Geometry: final body of the model. Coordinates: model frame, mm. A direction names the side the tool comes from. Give positions to 0.01 mm unless a question says otherwise; leave off trailing zeros. Write each loop counter-clockwise with the first axis right and the second up, starting at its lowest first coordinate (ties: lowest second). Pieces come first, ordered by that corner, then holes. Notation, with made-up numbers: (-10.75, -9.5) - (-4.75, -9.5) arc R28 cw to (-4.75, 18.5) - close; hole circle Ø10 at (35.5, 1). An arc over 180 degrees is marked (long way). Return JSON: item names as keys, results as strings.
from build123d import *

# Parameters (mm, degrees)
SKETCH1_R               = 4
BOSS_EXTRUDE1_DEPTH     = 20
CUT_EXTRUDE1_DEPTH      = 52
CUT_EXTRUDE1_DEPTH_BACK = 35
SKETCH2_W               = 10
SKETCH2_H               = 20
SKETCH3_W               = 10
SKETCH3_H               = 10
CUT_EXTRUDE2_DEPTH      = 52
CUT_EXTRUDE3_START      = -5
CUT_EXTRUDE3_DEPTH      = 10
CUT_EXTRUDE4_START      = -5
CUT_EXTRUDE4_DEPTH      = 10
FILLET1_R               = 2
SKETCH9_R               = 4
SKETCH9_R_2             = 2.5
BOSS_EXTRUDE2_DEPTH     = 3.5
BOSS_EXTRUDE3_START     = -3.5
SKETCH10_R              = 4
SKETCH10_R_2            = 2.5
BOSS_EXTRUDE3_DEPTH     = 3.5


with BuildPart() as part:
    # Sketch1 → Boss-Extrude1 (new body)
    with BuildSketch(Plane(origin=(0, 0, 0), x_dir=(0, 0, -1), z_dir=(1, 0, 0))):
        with BuildLine():
            Line((-41.59166249, 42.046001407), (58.40833751, 42.046001407))
            add(Edge.make_bspline(
                [(58.40833751, 42.046001407), (82.40833751, 34.546001407), (58.40833751, 27.046001407)],
                knots=[0, 0, 0, 1, 1, 1], degree=2))
            Line((58.40833751, 27.046001407), (-41.59166249, 27.046001407))
            add(Edge.make_bspline(
                [(-41.59166249, 42.046001407), (-61.59166249, 34.546001407), (-41.59166249, 27.046001407)],
                knots=[0, 0, 0, 1, 1, 1], degree=2))
        make_face()
        with Locations((60.40833751, 34.546001407)):
            Circle(SKETCH1_R, mode=Mode.SUBTRACT)
    extrude(amount=BOSS_EXTRUDE1_DEPTH)

    # Sketch2 → Cut-Extrude1 (cut, two sides: drawn at the far end of the back side and taken through both)
    with BuildSketch(Plane(origin=(0, 0, 0), x_dir=(1, 0, 0), z_dir=(0, 1, 0)).offset(-CUT_EXTRUDE1_DEPTH_BACK)):
        with Locations((10, 60.40833751)):
            Rectangle(SKETCH2_W, SKETCH2_H)
    extrude(amount=CUT_EXTRUDE1_DEPTH + CUT_EXTRUDE1_DEPTH_BACK, mode=Mode.SUBTRACT)

    # Sketch3 → Cut-Extrude2 (cut)
    with BuildSketch(Plane.XZ.offset(-27.046001407)):
        with Locations((10, 46.59166249)):
            Rectangle(SKETCH3_W, SKETCH3_H)
    extrude(amount=-CUT_EXTRUDE2_DEPTH, mode=Mode.SUBTRACT)

    # Sketch4 → Cut-Extrude3 (cut)
    with BuildSketch(Plane.ZY.offset(CUT_EXTRUDE3_START)):
        Polygon((-50.40833751, 34.546001407), (-50.40833751, 42.046001407), (-37.417956453, 42.046001407), align=None)
    extrude(amount=-CUT_EXTRUDE3_DEPTH, mode=Mode.SUBTRACT)

    # Sketch5 → Cut-Extrude4 (cut)
    with BuildSketch(Plane.ZY.offset(CUT_EXTRUDE4_START)):
        Polygon((-50.40833751, 27.046001407), (-50.40833751, 34.546001407), (-37.417956453, 27.046001407), align=None)
    extrude(amount=-CUT_EXTRUDE4_DEPTH, mode=Mode.SUBTRACT)

    # Fillet1
    fillet1_edges = [part.edges().sort_by_distance(p)[0] for p in [
        (10, 34.546001407, -50.40833751),
    ]]
    fillet(fillet1_edges, radius=FILLET1_R)

    # Sketch9 → Boss-Extrude2 (add)
    with BuildSketch(Plane.ZY):
        with Locations((-60.40833751, 34.546001407)):
            Circle(SKETCH9_R)
        with Locations((-60.40833751, 34.546001407)):
            Circle(SKETCH9_R_2, mode=Mode.SUBTRACT)
    extrude(amount=-BOSS_EXTRUDE2_DEPTH)

    # Sketch10 → Boss-Extrude3 (add)
    with BuildSketch(Plane(origin=(20, 0, 0), x_dir=(0, 0, -1), z_dir=(1, 0, 0)).offset(BOSS_EXTRUDE3_START)):
        with Locations((60.40833751, 34.546001407)):
            Circle(SKETCH10_R)
        with Locations(Location((60.40833751, 34.546001407, 0), (0, 0, 180))):
            Circle(SKETCH10_R_2, mode=Mode.SUBTRACT)
    extrude(amount=BOSS_EXTRUDE3_DEPTH)


solid = part.part
Q1. Set-up query: faces 1 (the cylindrical face through (4.24, 37.92, -62.56)), 2 (the flat face through (15, 34, 45)), 3 (the flat face through (9.93, 29.97, -42.48)), 4 (the flat face through (0, 35, -11)), 5 (the cylindrical face through (10.07, 34.52, -48.41)). Return all of +Z, -Z, +X, -X, +Y, -Y with unobstructed straight access to the full face (end or side cutting, diameter ignored); none if empty.
Answer key:
{"face 1": "none", "face 2": "+Z, +Y, -Y", "face 3": "-Z, -Y", "face 4": "+Z, -Z, -X, +Y, -Y", "face 5": "-Z"}
Q2. Section query A-A, the plane z = -54.5. Return the cut outline in (x, y).
Answer key:
{"outline": "(0, 27.05) - (5, 27.05) - (5, 42.05) - (0, 42.05) - close; (15, 27.05) - (20, 27.05) - (20, 42.05) - (15, 42.05) - close"}
Q3. Section query B-B, the plane x = 7.5. Return the cut outline in (y, z).
Answer key:
{"outline": "(27.05, -37.42) - (32.81, -47.41) arc R2 ccw to (36.28, -47.41) - (42.05, -37.42) - (42.05, 41.59) - (27.05, 41.59) - close"}
Q4. Mould query, pull axis Y, two halves, no side actions, for faces 6 (the cylindrical face through (15.74, 37.92, -62.56)), 7 (the flat face through (5, 34, 45)), 8 (the flat face through (9.93, 39.202, -42.343)). Classes: pulls with the +Y half, pulls with the -Y half, needs draft (parallel to the pull), parting line crosses it, or undercut.
Answer key:
{"face 6": "undercut", "face 7": "needs draft", "face 8": "pulls with the +Y half"}
Q5. Material intervals for probe 1 along X at (y, z) = (40.25, 44); probe 2 along Z at (x, y) = (17.75, 33.5); probe 3 along Y at (x, z) = (17.25, -59.5), sorted ascending. Write a range as [from, to].
Answer key:
{"probe 1": "x = [0, 5], [15, 20]", "probe 2": "z = [-70.17, -62.68], [-58.14, 51.4]", "probe 3": "y = [27.4, 32.22], [36.88, 41.7]"}
Q6. Pin query (flat end, axial travel): P1, Ø9, axis at y = 33.5, z = -61.5, coming from the -X side; P2, Ø8, axis at x = 9.5, y = 34.5, coming from the +Z side; P3, Ø3, axis at x = 15, y = 39.5, coming from the -Z side; P4, Ø5, axis at x = 10, z = -50.5, coming from the +Y side. Return the tip coordinate at first contact, or that it passes through.
Answer key:
{"P1": "stops at x = 0", "P2": "stops at z = 41.59", "P3": "stops at z = -67.86", "P4": "stops at y = 35.76"}
